Geometry check sheet. Reference: the model listing, model coordinates, mm. Face numbers are marked on the shaded views. Round coordinates to 2 decimals unless told otherwise and drop trailing zeros. Order: outer loops, then holes, each group sorted by start corner. A loop starts at its lowest first (then second) coordinate and runs counter-clockwise, first axis right, second up.
(1) Sectioned sample at A-A (z = 0). Record the boundary of the cut face in (x, y), plus the area to 3 significant figures.
(2) Material ranges on line 1 along Z through (x, y) = (16.5, 0.1); line 2 along X through (y, z) = (0.9, -2.1); line 3 along Z through (x, y) = (6.5, 2.05), recorded low to high.
(3) Release check for a two-part mould opening along X. For the marked faces 1 and 2 record: +X half, -X half, draft (parallel to the pull), parting line (faces both ways), or undercut.
(4) Go/stop test with flat-tipped pins: pin 1 (2 mm diameter, centred on x = 2, z = 2.5, fed in from +Y); pin 2 (1 mm diameter, centred on x = 21.5, z = -2, fed in from -Y); pin 3 (2 mm diameter, centred on x = -2.5, y = -2.5, fed in from -Z). Record where each tip stops, or that it passes through.
(5) Sectioned sample at C-C (x = 17). Record the boundary of the cut face in (y, z), plus the area to 3 significant figures.
Autodesk Inventor part; units mm, degrees
ref_plane "Work Plane1" through (2.75, 0, 0) normal (0, -1, 0) x (1, 0, 0)
ref_plane "YZ Plane" through (0, 0, 0) normal (1, 0, 0) x (0, 1, 0)
ref_plane "XZ Plane" through (0, 0, 0) normal (0, 1, 0) x (-1, 0, 0)
sketch "Szkic1" plane through (0, 0, 0) normal (0, 0, 1) x (1, 0, 0)
  line L0 (28, 3) -> (28, 0)
  line L1 (-6, 0) -> (28, 0)
  line L2 (-12.8, 0) -> (34.8, 0)
  line L3 (0, 3.6) -> (0, -0.6)
  line L4 (-6, 3) -> (-6, 0)
  line L5 (10, 3) -> (10, 0) construction
  line L6 (-12.8, 0) -> (34.8, 0)
  line L7 (-6, 3) -> (28, 3)
  dimension "d4" = 6
  dimension "d5" = 28
  dimension "d6" = 18
  dimension "d13" = 6
revolve "Bryła" add sketch "Szkic1" angle 360 about axis through (-6, 0, 0) along (1, 0, 0)
thread "Gwint1"
thread "Gwint2"
chamfer "Faza1" distance 1 angle 45 1 edges at (-6, -3, 0) measured on face at (16.6667, 2.9903, -0.2414)
chamfer "Faza2" distance 1 angle 45 1 edges at (28, -3, 0) measured on face at (6, 2.9612, -0.4812)
sketch "Sketch5" plane through (0, 0, 0) normal (0, 0, 1) x (1, 0, 0)
  line L0 (-5, 3) -> (27, 3)
  line L1 (-5, -3) -> (27, -3)
  line L2 (28, 2) -> (28, -2)
  line L3 (-6, -2) -> (-6, 2)
  line L4 (10, 3) -> (9.5, 2.5)
  line L5 (9.5, 2.5) -> (7.5, 3)
  line L6 (-12.8, 0) -> (34.8, 0)
  point P0 (0, 0)
  dimension "d87" = 45
  dimension "d90" = 18
  dimension "d91" = 0.5
  dimension "d92" = 2.5
revolve "IDS_REVOLUTION{1}" cut sketch "Sketch5" angle 360 about axis through (-10, 0, 0) along (1, 0, 0)
sketch "Sketch6" plane through (0, 0, 0) normal (0, 0, 1) x (1, 0, 0)
  line L0 (-5, 3) -> (7.5, 3)
  line L1 (-6, -2) -> (-6, 2)
  line L2 (-1.25, 3) -> (-0.75, 2.5)
  line L3 (-0.75, 2.5) -> (0, 3)
  line L4 (-8.7, 0) -> (10.2, 0)
  point P0 (0, 0)
  dimension "d94" = 45
  dimension "d95" = 6
  dimension "d96" = 0.5
  dimension "d97" = 1.25
revolve "IDS_REVOLUTION{2}" cut sketch "Sketch6" angle 360 about axis through (-10, 0, 0) along (1, 0, 0)
ref_plane "Work Plane1" through (2.75, 0, 0) normal (0, -1, 0) x (1, 0, 0)
equation "\"d4\" = KOH"
equation "\"d5\" = NLG"
equation "\"d6\" = GEL"
equation "\"d13\" = GD"
equation "\"d1\" = KOH"
equation "\"d7\" = GEL"
equation "\"d9\" = -0.5 * SPD + 0.5 * GD"
equation "\"d10\" = -0.5 * SPD + 0.5 * GD"
equation "\"d11\" = -0.5 * SPD + 0.5 * GD"
equation "\"d12\" = -0.5 * SPD + 0.5 * GD"
equation "\"d90\" = GEL"
equation "\"d91\" = -0.25 * SPD + 0.25 * GD"
equation "\"d92\" = X1"
equation "\"d95\" = KOH"
equation "\"d96\" = -0.25 * SPD + 0.25 * GD"
equation "\"d97\" = X2"
equation "\"NLG\" = 28"
equation "\"GEL\" = 18"
equation "\"GAL\" = 0.61345 * PTC"
equation "\"SPD\" = 4"
equation "\"d0\" = GD"
equation "\"GUL\" = 0.61345 * PTC"
equation "\"KOH\" = 6"
equation "\"GD\" = 6"
equation "\"BDM\" = NND"
equation "\"GUL1\" = GUL"
equation "\"GAL1\" = GAL"
equation "\"d80\" = -GUL - GEL"
equation "\"d86\" = -KOH + GUL1"
equation "\"X1\" = 2.5"
equation "\"X2\" = 1.25"
equation "\"PTC\" = 1"
equation "\"THREADDIA\" = 6"
equation "\"TOA\" = 30deg"
equation "\"NND\" = 6"
equation "\"GD1\" = THREADDIA - 1.2269 * PTC"
properties part number "DIN 938 - M6 x 28" material "Stal, miękka"
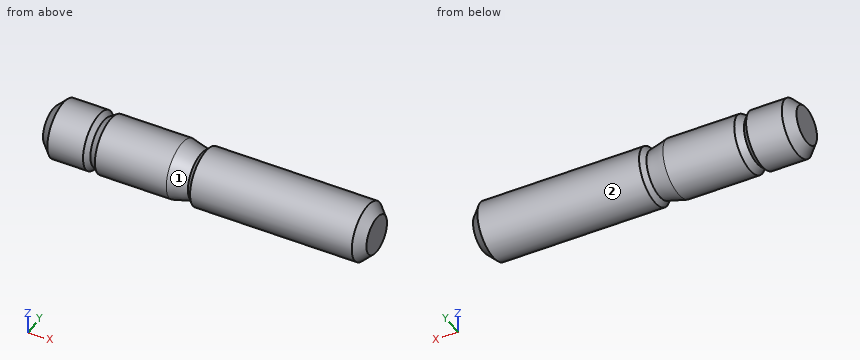
Answer below:
1. outline: (-6, -2) - (-5, -3) - (-1.25, -3) - (-0.75, -2.5) - (0, -3) - (7.5, -3) - (9.5, -2.5) - (10, -3) - (27, -3) - (28, -2) - (28, 2) - (27, 3) - (10, 3) - (9.5, 2.5) - (7.5, 3) - (0, 3) - (-0.75, 2.5) - (-1.25, 3) - (-5, 3) - (-6, 2) - close
1. area: 200 mm2
2. line 1: z = -3 to 3
2. line 2: x = -5.72 to 27.72
2. line 3: z = -2.19 to 2.19
3. face 1: undercut
3. face 2: draft
4. pin 1: stops at y = 2.6
4. pin 2: stops at y = -2.6
4. pin 3: stops at z = -2.6
5. outline: circle Ø6 at (0, 0)
5. area: 28.3 mm2
